Model file for the job. Use its own axes, mm. A direction names the side the tool comes from. Round coordinates to 2 decimals unless told otherwise and drop trailing zeros. Loops run counter-clockwise (first coordinate to the right, second up) from the corner with the lowest first, then second, coordinate; pieces in that order, holes last. Notation, with made-up numbers: (-23, -10.75) -> (26, -10.75) arc R10 cw to (26, 2.25) -> close; hole circle Ø3 at (-35, 83). An arc over 180 degrees is marked (long way). Use a Markdown table: item, result. Add a question column.
```python
from build123d import *

# Parameters (mm, degrees)
F1_DEPTH  = 12.5
F3_DEPTH  = 25
F4_R      = 9.05
F5_DEPTH  = 55
F6_R      = 9.15
F7_DEPTH  = 52.5
F9_DEPTH  = 57.501
F11_DEPTH = 25
F13_DEPTH = 1


with BuildPart() as f1:
    # F0 (on Top) → F1 (new body, symmetric)
    with BuildSketch(Plane.XY):
        with BuildLine():
            ThreePointArc((50, 0), (0, -50), (-50, 0))
            Line((-50, 0), (-55, 0))
            ThreePointArc((-55, 0), (0, -55), (55, 0))
            Line((55, 0), (50, 0))
        make_face()
    extrude(amount=F1_DEPTH, both=True)

    # F2 (on face) → F3 (join)
    with BuildSketch(Plane.XY.offset(12.5)):
        with BuildLine():
            ThreePointArc((55, 0), (0, -55), (-55, 0))
            Line((-55, 0), (-55, -57.5))
            Line((-55, -57.5), (0, -57.5))
            Line((0, -57.5), (55, -57.5))
            Line((55, -57.5), (55, 0))
        make_face()
    extrude(amount=-F3_DEPTH)

    # F4 (on Front) → F5 (cut)
    with BuildSketch(Plane.XZ):
        Circle(F4_R)
    extrude(amount=F5_DEPTH, mode=Mode.SUBTRACT)

    # F6 (on Right) → F7 (cut, symmetric)
    with BuildSketch(Plane.YZ):
        with Locations((-11, 0)):
            Circle(F6_R)
    extrude(amount=F7_DEPTH, both=True, mode=Mode.SUBTRACT)

    # F8 (on face) → F9 (cut, through all)
    with BuildSketch(Plane.XZ.offset(57.5)):
        Polygon((15, 12.5), (-15, 12.5), (-15, 48.375133), (-89.987703, 48.375133), (-91.230497, -54.7974), (-15, -56.857262), (-15, -12.5), (15, -12.5), (15, -3), (21, -3), (21, 0), (21, 3), (15, 3), align=None)
    extrude(amount=-F9_DEPTH, mode=Mode.SUBTRACT)

    # F10 (on face) → F11 (cut)
    with BuildSketch(Plane(origin=(0, 0, -12.5), x_dir=(1, 0, 0), z_dir=(0, 0, -1))):
        Polygon((50, 27.5), (50, 52.5), (25, 52.5), align=None)
    extrude(amount=-F11_DEPTH, mode=Mode.SUBTRACT)

    # F12 (on face) → F13 (join)
    with BuildSketch(Plane(origin=(0, 0, -12.5), x_dir=(1, 0, 0), z_dir=(0, 0, -1))):
        with BuildLine():
            Line((16.194436, 57.5), (16.194436, 58.579612))
            ThreePointArc((16.194436, 58.579612), (14.941014, 76.499807), (13.922594, 58.564722))
            Line((13.922594, 58.564722), (15, 57.5))
            Line((15, 57.5), (16.194436, 57.5))
        make_face()
        with BuildLine():
            Line((55, 56.879111), (56.230159, 57.5))
            ThreePointArc((56.230159, 57.5), (71.021188, 67.707692), (55.175651, 59.228867))
            Line((55.175651, 59.228867), (54.298293, 57.5))
            Line((54.298293, 57.5), (55, 57.5))
            Line((55, 57.5), (55, 56.879111))
        make_face()
        with BuildLine():
            Line((53.94445, 0), (54.919557, -1.423379))
            ThreePointArc((54.919557, -1.423379), (66.865014, -14.838437), (56.741846, 0))
            Line((56.741846, 0), (55, 1.024423))
            Line((55, 1.024423), (55, 0))
            Line((55, 0), (53.94445, 0))
        make_face()
    extrude(amount=-F13_DEPTH)


solid = f1.part
```
1) Pin check, flat tips, straight feed: pin 1 Ø7.5 at (x, z) = (36, 4.5) entering from +Y; pin 2 Ø1.5 at (y, z) = (-34, 3) entering from -X; pin 3 Ø14.5 at (y, z) = (-14.5, 0.5) entering from -X. Stop position of each tip, or through.
2) Cut at D-D on y = -11. Write the cut outline in (x, z) (3 decimals), and give its area (3 significant figures).
3) Cut at A-A on x = 47.5. Write the cut outline in (y, z), and give its area (3 significant figures).
4) Pull direction Y, two halves, no side cores. Call faces 5 (the face through (36.074, -34.622, 0.175)), 6 (the face through (18, -52, 3)), 7 (the face through (37.3, -40.2, -0.2)), 8 (the face through (15.321, -76.494, -12.007)): +Y half, -Y half, draft (parallel to the pull), parting line (faces both ways), or undercut.
5) Wall check: probe 1 along Z at (x, y) = (49.5, -11); probe 2 along Y at (x, z) = (50.5, 0); probe 3 along Z at (x, y) = (53, 10). Give the ranges that are in metal, low to high. Write a range as from..to.
6) Cut at C-C on y = -61.5. Write the cut outline in (x, z), and give its area (3 significant figures).
7) Cut at B-B on z = 10.75. Write the cut outline in (x, y), and give its area (3 significant figures).
8) Tool access for faces 1 (the face through (38, -52.5, 0)), 2 (the face through (49.93, -20.14, 0.4)), 3 (the face through (18, -52, -3)), 4 (the face through (15, -67, -11.5)): list every direction of +Z, -Z, +X, -X, +Y, -Y with a clear straight run to the whole face (end or side of a thin tool).
Established:
| question | item | result |
|---|---|---|
| 1 | pin 1 | stops at y = -30.33 |
| 1 | pin 2 | stops at x = 35.95 |
| 1 | pin 3 | stops at x = 45.02 |
| 2 | outline | (48.775, -12.5) -> (55, -12.5) -> (55, 12.5) -> (48.775, 12.5) -> (48.775, 9.15) -> (52.5, 9.15) -> (52.5, -9.15) -> (48.775, -9.15) -> close |
| 2 | area | 87.5 mm^2 |
| 3 | outline | (-57.5, -12.5) -> (-52.5, -12.5) -> (-52.5, 12.5) -> (-57.5, 12.5) -> close; (-30, -12.5) -> (-15.61, -12.5) -> (-15.61, -7.9) arc R9.15 cw to (-15.61, 7.9) -> (-15.61, 12.5) -> (-30, 12.5) -> close |
| 3 | area | 434 mm^2 |
| 4 | face 5 | +Y half |
| 4 | face 6 | draft |
| 4 | face 7 | undercut |
| 4 | face 8 | undercut |
| 5 | probe 1 | z = -12.5..-9.15, 9.15..12.5 |
| 5 | probe 2 | y = -57.5..-20.15, -1.85..0 |
| 5 | probe 3 | z = -12.5..-11.5 |
| 6 | outline | (8.29, -12.5) -> (21.71, -12.5) -> (21.71, -11.5) -> (8.29, -11.5) -> close; (54.47, -12.5) -> (72.21, -12.5) -> (72.21, -11.5) -> (54.47, -11.5) -> close |
| 6 | area | 31.2 mm^2 |
| 7 | outline | (15, -57.5) -> (55, -57.5) -> (55, 0) -> (50, 0) arc R50 cw to (15, -47.7) -> close; hole (25, -52.5) -> (50, -52.5) -> (50, -27.5) -> close |
| 7 | area | 763 mm^2 |
| 8 | face 1 | +Z, -Z |
| 8 | face 2 | -X |
| 8 | face 3 | -X, +Y, -Y |
| 8 | face 4 | +Z, +X, -X, -Y |
